Geometry check sheet. Reference: the model listing, model coordinates, mm. Coordinates: 2 decimals unless noted, no trailing zeros. Loops run counter-clockwise (first coordinate to the right, second up) from the corner with the lowest first, then second, coordinate; pieces in that order, holes last.
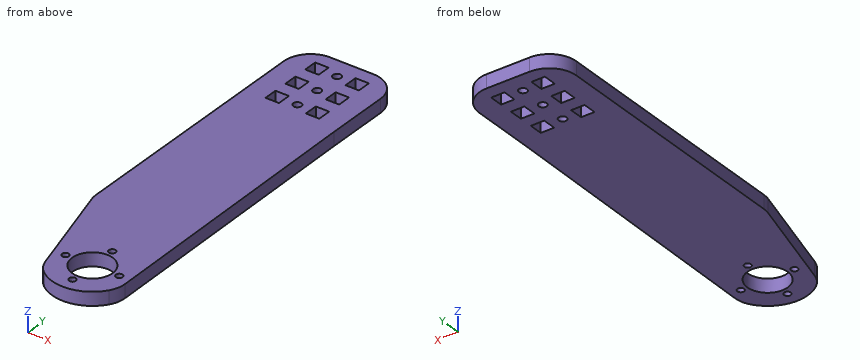
from build123d import *

# Parameters (mm, degrees)
SKETCH1_R           = 7.5
SKETCH1_R_2         = 1.25
SKETCH1_R_3         = 1.5
SKETCH1_W           = 5
SKETCH1_H           = 5
BOSS_EXTRUDE1_DEPTH = 5
FILLET1_R           = 10
FILLET2_R           = 10


with BuildPart() as part:
    # Sketch1 → Boss-Extrude1 (new body)
    with BuildSketch(Plane.XY):
        with BuildLine():
            Line((0, 44.138584039), (10.984892076, 3.520179201))
            ThreePointArc((10.984892076, 3.520179201), (25.289734382, -2.324207111), (37.164554201, 7.563867476))
            Line((37.164554201, 7.563867476), (36, 116.603941586))
            Line((36, 116.603941586), (36, 150))
            Line((36, 150), (0, 150))
            Line((0, 150), (0, 44.138584039))
        make_face()
        with Locations((23, 12.5)):
            Circle(SKETCH1_R, mode=Mode.SUBTRACT)
        with Locations((23, 22.5)):
            Circle(SKETCH1_R_2, mode=Mode.SUBTRACT)
        with Locations((13, 12.5)):
            Circle(SKETCH1_R_2, mode=Mode.SUBTRACT)
        with Locations((23, 2.5)):
            Circle(SKETCH1_R_2, mode=Mode.SUBTRACT)
        with Locations((33, 12.5)):
            Circle(SKETCH1_R_2, mode=Mode.SUBTRACT)
        with Locations((18, 142.5)):
            Circle(SKETCH1_R_3, mode=Mode.SUBTRACT)
        with Locations((18, 122.5)):
            Circle(SKETCH1_R_3, mode=Mode.SUBTRACT)
        with Locations((18, 132.5)):
            Circle(SKETCH1_R_3, mode=Mode.SUBTRACT)
        with Locations((10.5, 142.5)):
            Rectangle(SKETCH1_W, SKETCH1_H, mode=Mode.SUBTRACT)
        with Locations((25.5, 142.5)):
            Rectangle(SKETCH1_W, SKETCH1_H, mode=Mode.SUBTRACT)
        with Locations((10.5, 122.5)):
            Rectangle(SKETCH1_W, SKETCH1_H, mode=Mode.SUBTRACT)
        with Locations((25.5, 122.5)):
            Rectangle(SKETCH1_W, SKETCH1_H, mode=Mode.SUBTRACT)
        with Locations((10.5, 132.5)):
            Rectangle(SKETCH1_W, SKETCH1_H, mode=Mode.SUBTRACT)
        with Locations((25.5, 132.5)):
            Rectangle(SKETCH1_W, SKETCH1_H, mode=Mode.SUBTRACT)
    extrude(amount=BOSS_EXTRUDE1_DEPTH)

    # Fillet1
    fillet1_edges = [part.edges().sort_by_distance(p)[0] for p in [
        (0, 150, 2.5),
        (36, 150, 2.5),
    ]]
    fillet(fillet1_edges, radius=FILLET1_R)

    # Fillet2
    fillet2_edges = [part.edges().sort_by_distance(p)[0] for p in [
        (10.984892076, 3.520179201, 2.5),
        (0, 44.138584039, 2.5),
        (36, 116.603941586, 2.5),
        (37.164554201, 7.563867476, 2.5),
    ]]
    fillet(fillet2_edges, radius=FILLET2_R)


solid = part.part
(1) Scan lines: L1, parallel to X at y = 132.5, z = 2.8; L2, parallel to Y at x = 17, z = 1.3; L3, parallel to X at y = 121.5, z = 2.6. Record each from-to range of solid material in increasing order.
Findings:
L1: x = 0 to 8, 13 to 16.5, 19.5 to 23, 28 to 36
L2: y = -1.25 to 8, 17 to 121.38, 123.62 to 131.38, 133.62 to 141.38, 143.62 to 150
L3: x = 0 to 8, 13 to 16.88, 19.12 to 23, 28 to 36
(2) Sectioned sample at C-C on z = 2.1. State how many separate pieces and enclosed holes the cut face has, and give its area (3 significant figures).
Findings:
separate pieces: 1
enclosed holes: 14
area: 4,800 mm2
(3) Gauge pin test, flat ends, axial feed: pin 1 Ø3 at (y, z) = (21.5, 2.5) entering from +X; pin 2 Ø2.5 at (y, z) = (132.5, 3.5) entering from +X; pin 3 Ø2.5 at (x, z) = (26.5, 1.5) entering from -Y; pin 4 Ø5 at (x, y) = (18, 122.5) entering from +Z. Record the tip position at first contact, or that the pin passes through.
Findings:
pin 1: stops at x = 37.03
pin 2: stops at x = 36
pin 3: stops at y = -2.33
pin 4: stops at z = 5
(4) Sectioned sample at A-A on y = 132.5. Record the cut outline in (x, z).
Findings:
outline: (0, 0) - (8, 0) - (8, 5) - (0, 5) - close; (13, 0) - (16.5, 0) - (16.5, 5) - (13, 5) - close; (19.5, 0) - (23, 0) - (23, 5) - (19.5, 5) - close; (28, 0) - (36, 0) - (36, 5) - (28, 5) - close
(5) Sectioned sample at D-D on y = 63.5. Record the cut outline in (x, z).
Findings:
outline: (0, 0) - (36.57, 0) - (36.57, 5) - (0, 5) - close
(6) Sectioned sample at B-B on x = 18. Record the cut outline in (y, z).
Findings:
outline: (-1.64, 0) - (6.91, 0) - (6.91, 5) - (-1.64, 5) - close; (18.09, 0) - (121, 0) - (121, 5) - (18.09, 5) - close; (124, 0) - (131, 0) - (131, 5) - (124, 5) - close; (134, 0) - (141, 0) - (141, 5) - (134, 5) - close; (144, 0) - (150, 0) - (150, 5) - (144, 5) - close
